Part model, mm, in its own coordinate system. A direction names the side the tool comes from. Coordinates: 2 decimals unless noted, no trailing zeros. Write each loop counter-clockwise with the first axis right and the second up, starting at its lowest first coordinate (ties: lowest second). Pieces come first, ordered by that corner, then holes. Notation, with made-up numbers: (-38.75, -31) - (-34.75, -31) arc R23 ccw to (-34.75, -5) - close; hole circle Ø8 at (30.25, -23.5). An arc over 180 degrees is marked (long way). Use a Markdown table: item, result.
```python
from build123d import *

# Parameters (mm, degrees)
SKETCH_1_W             = 50.5
SKETCH_1_H             = 4.5
EXTRUDE_1_DEPTH        = 2.5
EXTRUDE_START          = -4
SKETCH_2_R             = 0.4
EXTRUDE_2_DEPTH        = 10
PATTERN_LINEAR_2_COUNT = 20
PATTERN_LINEAR_2_PITCH = 2.54
FILLET_1_R             = 1


with BuildPart() as part:
    # ｽｹｯﾁ1 → ﾎﾞｽ - 押し出し1 (new body)
    with BuildSketch(Plane.XY):
        Rectangle(SKETCH_1_W, SKETCH_1_H)
    extrude(amount=EXTRUDE_1_DEPTH)

    # ｽｹｯﾁ2 → ﾎﾞｽ - 押し出し2 (add)
    with BuildSketch(Plane.XY.offset(2.5).offset(EXTRUDE_START)):
        with Locations((-24.25, 1.37)):
            Circle(SKETCH_2_R)
        with Locations((-24.25, -1.17)):
            Circle(SKETCH_2_R)
    extrude_2 = extrude(amount=EXTRUDE_2_DEPTH)

    # 直線ﾊﾟﾀｰﾝ2: ﾎﾞｽ - 押し出し2 ×20
    with Locations(*[(i * PATTERN_LINEAR_2_PITCH, 0, 0) for i in range(1, PATTERN_LINEAR_2_COUNT)]):
        add(extrude_2)

    # ﾌｨﾚｯﾄ1
    fillet_1_edges = [part.edges().sort_by_distance(p)[0] for p in [
        (25.25, -2.25, 1.25),
        (-25.25, -2.25, 1.25),
        (-25.25, 2.25, 1.25),
        (25.25, 2.25, 1.25),
    ]]
    fillet(fillet_1_edges, radius=FILLET_1_R)


solid = part.part
```
Item 1: Drill centre lines: probe 1 along Y at (x, z) = (-4, 7.75); probe 2 along Z at (x, y) = (10.5, -1.6); probe 3 along Y at (x, z) = (-16.5, 8). Where is each one in solid material? Low to high.
From the geometry:
| item | result |
|---|---|
| probe 1 | -1.56 to -0.78, 0.98 to 1.76 |
| probe 2 | 0 to 2.5 |
| probe 3 | -1.55 to -0.79, 0.99 to 1.75 |
Item 2: Band-saw the part on C-C, the plane y = -0.3. Give the cut face in (x, z).
From the geometry:
| item | result |
|---|---|
| outline | (-25.25, 0) - (25.25, 0) - (25.25, 2.5) - (-25.25, 2.5) - close |
Item 3: Which spindle directions (+Z, -Z, +X, -X, +Y, -Y) get a long thin tool onto all of the face, cutting with end or side? Do faces 1 (the face through (25.25, 0, 1)), 2 (the face through (8.37, 1.39, 5.46)), 3 (the face through (-13.71, -1.05, -0.76)). Say none if no direction does.
From the geometry:
| item | result |
|---|---|
| face 1 | +Z, -Z, +X, +Y, -Y |
| face 2 | +Z |
| face 3 | -Z |
Item 4: Band-saw the part on B-B, the plane x = -10. Give the cut face in (y, z).
From the geometry:
| item | result |
|---|---|
| outline | (-2.25, 0) - (2.25, 0) - (2.25, 2.5) - (-2.25, 2.5) - close |
Item 5: Two-plate mould, pull along X, no slides. Class faces 4 (the face through (-9.41, -1.15, -0.76)), 5 (the face through (-24.965, 1.949, 1.268)), 6 (the face through (24.949, -1.965, 1.268)): pulls with the +X half, pulls with the -X half, needs draft (parallel to the pull), parting line crosses it, or undercut.
From the geometry:
| item | result |
|---|---|
| face 4 | undercut |
| face 5 | pulls with the -X half |
| face 6 | pulls with the +X half |
Item 6: Band-saw the part on A-A, the plane z = 7. Count the separate pieces of the cut face and the enclosed holes in it, then the cut area to 3 significant figures.
From the geometry:
| item | result |
|---|---|
| separate pieces | 40 |
| enclosed holes | 0 |
| area | 20.1 mm^2 |
